```python
from build123d import *

# Parameters (mm, degrees)
SKETCH_1_W      = 4
SKETCH_1_H      = 4
EXTRUDE_1_DEPTH = 6
SKETCH_2_R      = 2
EXTRUDE_2_DEPTH = 49
CHAMFER_1_SIZE  = 0.5
CHAMFER_2_SIZE  = 0.2
FILLET_1_R      = 0.1


with BuildPart() as part:
    # 草图1 → 凸台-拉伸1 (new body)
    with BuildSketch(Plane(origin=(0, 0, 0), x_dir=(0, 0, -1), z_dir=(1, 0, 0))):
        Rectangle(SKETCH_1_W, SKETCH_1_H)
    extrude(amount=EXTRUDE_1_DEPTH)

    # 草图2 → 凸台-拉伸2 (add)
    with BuildSketch(Plane(origin=(6, 0, 0), x_dir=(0, 0, -1), z_dir=(1, 0, 0))):
        Circle(SKETCH_2_R)
    extrude(amount=EXTRUDE_2_DEPTH)

    # 倒角1
    chamfer_1_edges = [part.edges().sort_by_distance(p)[0] for p in [
        (55, 0, 2),
    ]]
    chamfer(chamfer_1_edges, length=CHAMFER_1_SIZE)

    # 倒角2
    chamfer_2_edges = [part.edges().sort_by_distance(p)[0] for p in [
        (0, 0, 2),
        (0, 2, 0),
        (0, 0, -2),
        (0, -2, 0),
    ]]
    chamfer(chamfer_2_edges, length=CHAMFER_2_SIZE)

    # 圆角1
    fillet_1_edges = [part.edges().sort_by_distance(p)[0] for p in [
        (3.1, -2, 2),
        (3.1, 2, 2),
        (3.1, 2, -2),
        (3.1, -2, -2),
    ]]
    fillet(fillet_1_edges, radius=FILLET_1_R)


solid = part.part
```
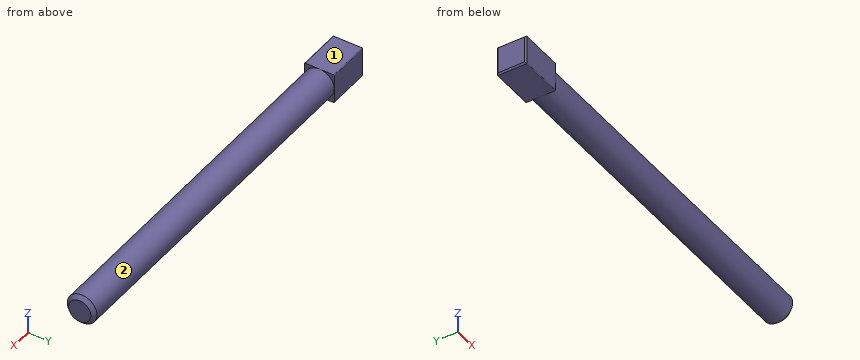
For this review, take the finished solid that the model builds, in its own axes (mm). Face numbers are marked on the shaded views. A direction names the side the tool comes from. Round coordinates to 2 decimals unless told otherwise and drop trailing zeros. Order: outer loops, then holes, each group sorted by start corner. A loop starts at its lowest first (then second) coordinate and runs counter-clockwise, first axis right, second up. Notation, with made-up numbers: (47.25, 4.25) -> (105.25, 4.25) arc R8 cw to (105.25, 19.25) -> close; hole circle Ø8 at (69.25, 5). An arc over 180 degrees is marked (long way). Use a Markdown table: item, result.
Item 1: For line 1 along X through (y, z) = (-1.8, -1.25); line 2 along Y through (x, z) = (6, 0.2); line 3 along Z through (x, y) = (9, -1.1), list the stretches that pass through material, from the lowest coordinate up. Write a range as [from, to].
Resolved:
| item | result |
|---|---|
| line 1 | x = [0, 6] |
| line 2 | y = [-1.99, 1.99] |
| line 3 | z = [-1.67, 1.67] |
Item 2: For pin 1 (1 mm diameter, centred on x = 24.5, z = 1, fed in from +Y); pin 2 (1 mm diameter, centred on y = -1.5, z = -1.5, fed in from +X); pin 3 (1 mm diameter, centred on x = 46, y = 1.5, fed in from -Z), all flat-tipped, find the tip position at first contact; note any pin that passes through.
Resolved:
| item | result |
|---|---|
| pin 1 | stops at y = 1.94 |
| pin 2 | stops at x = 54.88 |
| pin 3 | stops at z = -1.73 |
Item 3: Take a section at A-A (x = 38.5). State the section outline as (y, z) points, plus the area to 3 significant figures.
Resolved:
| item | result |
|---|---|
| outline | circle Ø4 at (0, 0) |
| area | 12.6 mm² |
Item 4: Machinability: for the marked faces 1 and 2, which of the approach directions +Z, -Z, +X, -X, +Y, -Y give a long, thin tool a straight path to every point of the face, cutting with its end or side? Answer none if there is none.
Resolved:
| item | result |
|---|---|
| face 1 | +Z, +X, -X, +Y, -Y |
| face 2 | +X |
